Source: CAD feature listing. Evaluate the final solid. Frame: model axes, mm. A direction names the side the tool comes from. Coordinates: 2 decimals unless noted, no trailing zeros. Loops run counter-clockwise (first coordinate to the right, second up) from the corner with the lowest first, then second, coordinate; pieces in that order, holes last. Notation, with made-up numbers: (61, 13) - (106, 13) arc R37 ccw to (106, 51) - close; hole circle Ø10 at (59, -15.5). An arc over 180 degrees is marked (long way). Use one line per item in the form item = value. Start each with the question number.
from build123d import *

# Parameters (mm, degrees)
SKETCH_3_R          = 2.5
CUT_EXTRUDE_1_DEPTH = 15
CUT_EXTRUDE_START   = -15
SKETCH_4_R          = 2.5
CUT_EXTRUDE_2_DEPTH = 15
CHAMFER_1_SIZE      = 0.5
CUT_EXTRUDE_3_DEPTH = 15


with BuildPart() as part:
    # 草图1 → 旋转1 (revolve)
    with BuildSketch(Plane(origin=(0, 0, 0), x_dir=(0, 0, -1), z_dir=(1, 0, 0)), mode=Mode.PRIVATE) as revolve_1_sk:
        with BuildLine():
            Line((0, 0), (0, 42.5))
            Line((0, 42.5), (40, 42.5))
            ThreePointArc((40, 42.5), (45.865854451, 40.631649689), (51.989578808, 40))
            Line((51.989578808, 40), (407.010421192, 40))
            ThreePointArc((407.010421192, 40), (413.134145549, 40.631649689), (419, 42.5))
            Line((419, 42.5), (454, 42.5))
            Line((454, 42.5), (454, 45))
            Line((454, 45), (555, 45))
            Line((555, 45), (555, 49))
            Line((555, 49), (563, 49))
            Line((563, 49), (563, 0))
            Line((563, 0), (0, 0))
        make_face()
    revolve(revolve_1_sk.sketch.rotate(Axis((0, 0, 0), (0, 0, 1)), 90), axis=Axis((0, 0, 0), (0, 0, 1)))

    # 草图2 → 切除-旋转1 (revolve, cut)
    with BuildSketch(Plane(origin=(0, 0, 0), x_dir=(0, 0, -1), z_dir=(1, 0, 0)), mode=Mode.PRIVATE) as cut_revolve_1_sk:
        Polygon((0, 0), (0, 34), (26, 34), (26, 30), (537, 30), (537, 34), (563, 34), (563, 0), align=None)
    revolve(cut_revolve_1_sk.sketch.rotate(Axis((0, 0, 0), (0, 0, 1)), 90), axis=Axis((0, 0, 0), (0, 0, 1)), mode=Mode.SUBTRACT)

    # 草图3 → 切除-拉伸1 (cut)
    with BuildSketch(Plane.XY):
        with Locations((0, 38)):
            Circle(SKETCH_3_R)
        with Locations((26.870057685, 26.870057685)):
            Circle(SKETCH_3_R)
        with Locations((38, 0)):
            Circle(SKETCH_3_R)
        with Locations((26.870057685, -26.870057685)):
            Circle(SKETCH_3_R)
        with Locations((0, -38)):
            Circle(SKETCH_3_R)
        with Locations((-26.870057685, -26.870057685)):
            Circle(SKETCH_3_R)
        with Locations((-38, 0)):
            Circle(SKETCH_3_R)
        with Locations((-26.870057685, 26.870057685)):
            Circle(SKETCH_3_R)
    extrude(amount=-CUT_EXTRUDE_1_DEPTH, mode=Mode.SUBTRACT)

    # 草图4 → 切除-拉伸2 (cut)
    with BuildSketch(Plane(origin=(0, 0, -563), x_dir=(-1, 0, 0), z_dir=(0, 0, -1)).offset(CUT_EXTRUDE_START)):
        with Locations(Location((0, 38, 0), (0, 0, 180))):
            Circle(SKETCH_4_R)
        with Locations(Location((26.870057685, 26.870057685, 0), (0, 0, 180))):
            Circle(SKETCH_4_R)
        with Locations(Location((38, 0, 0), (0, 0, 180))):
            Circle(SKETCH_4_R)
        with Locations(Location((26.870057685, -26.870057685, 0), (0, 0, 180))):
            Circle(SKETCH_4_R)
        with Locations(Location((0, -38, 0), (0, 0, 180))):
            Circle(SKETCH_4_R)
        with Locations(Location((-26.870057685, -26.870057685, 0), (0, 0, 180))):
            Circle(SKETCH_4_R)
        with Locations(Location((-38, 0, 0), (0, 0, 180))):
            Circle(SKETCH_4_R)
        with Locations(Location((-26.870057685, 26.870057685, 0), (0, 0, 180))):
            Circle(SKETCH_4_R)
    extrude(amount=CUT_EXTRUDE_2_DEPTH, mode=Mode.SUBTRACT)

    # 倒角1
    chamfer_1_edges = [part.edges().sort_by_distance(p)[0] for p in [
        (45, 0, -454),
        (49, 0, -563),
        (34, 0, 0),
        (34, 0, -563),
        (42.5, 0, 0),
    ]]
    chamfer(chamfer_1_edges, length=CHAMFER_1_SIZE)

    # 草图5 → 切除-拉伸3 (cut)
    with BuildSketch(Plane(origin=(0, 42.5, 0), x_dir=(1, 0, 0), z_dir=(0, 1, 0))):
        with BuildLine():
            Line((-2.5, 454), (-2.5, 469.5))
            ThreePointArc((-2.5, 469.5), (0, 472), (2.5, 469.5))
            Line((2.5, 469.5), (2.5, 454))
            Line((2.5, 454), (-2.5, 454))
        make_face()
    extrude(amount=CUT_EXTRUDE_3_DEPTH, mode=Mode.SUBTRACT)


solid = part.part
(1) Mould query, pull axis Y, two halves, no side actions, for faces 1 (the face through (-40.537, -12.766, -436.745)), 2 (the face through (36, 23, -454)), 3 (the face through (-16.128, -25.296, -285.077)). Classes: +Y half, -Y half, draft (parallel to the pull), parting line (faces both ways), or undercut.
(2) Material intervals for line 1 (X direction, y = 2, z = -280.5); line 2 (Y direction, x = -1, z = -245); line 3 (Y direction, x = 21.5, z = -286), sorted ascending.
(3) Cut plane A-A, the plane z = -155.5. Output: boundary loops of the cut face in (x, y).
(4) Access query for faces 4 (the face through (4.43, -33.71, -13.43)), 5 (the face through (39.96, -1.76, -231.99)), 6 (the face through (2.4, 30.1, -537)), 7 (the face through (11, -33, -563)), 8 (the face through (-46.737, -14.718, -558.802)). Directions: +Z, -Z, +X, -X, +Y, -Y. A direction counts if a zero-diameter tool reaches every point of the face in a straight line with its end or side. Return the directions, or none.
(5) Contact query for flat-ended pins moving along their axis: pin 1 (2 mm diameter, centred on y = -31.5, z = -478, fed in from -X); pin 2 (6 mm diameter, centred on y = 18, z = -210.5, fed in from -X); pin 3 (2.5 mm diameter, centred on x = 0.5, y = -38.5, fed in from -Z). Output: stop coordinate, or through.
Recorded:
q1.face_1 = parting line
q1.face_2 = draft
q1.face_3 = undercut
q2.line_1 = -39.95 to -29.93, 29.93 to 39.95
q2.line_2 = -39.99 to -29.98, 29.98 to 39.99
q2.line_3 = -33.73 to -20.92, 20.92 to 33.73
q3.outline = circle Ø80 at (0, 0); hole circle Ø60 at (0, 0)
q4.face_4 = +Z
q4.face_5 = none
q4.face_6 = -Z
q4.face_7 = -Z, +X, -X, +Y, -Y
q4.face_8 = +Z, -Z
q5.pin_1 = -33.09
q5.pin_2 = -37.08
q5.pin_3 = -548
